For this review, use the dimensioned drawing (mm, ordinates from the lowest corner) and the shaded views. Round coordinates to 2 decimals unless told otherwise and drop trailing zeros. Loops run counter-clockwise (first coordinate to the right, second up) from the corner with the lowest first, then second, coordinate; pieces in that order, holes last. Notation, with made-up numbers: (-9, 35.25) -> (46, 35.25) arc R28 cw to (46, 55.25) -> close; hole circle Ø5 at (-31, -31.5). An arc over 180 degrees is marked (long way). Use one line per item in the form item = value. Start each with the question number.
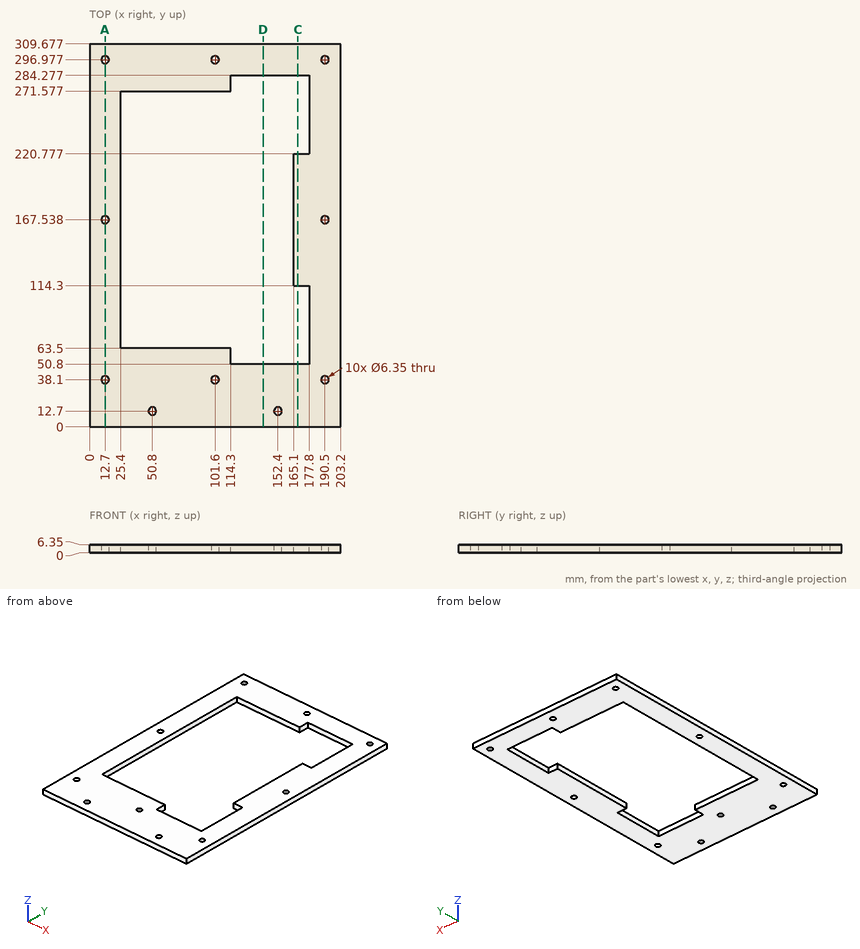
Item 1: Take a section at D-D on x = 140.5. Give the boundary of the cut face in (y, z), plus the area to 3 significant figures.
Item 2: Wall thickness on line 1 (Y direction, x = 190, z = 1) (1 decimal); line 2 (Y direction, x = 152.4, z = 4.25) (1 decimal); line 3 (Y direction, x = 101.6, z = 4.25) (1 decimal): over which ranges is each line inside the solid? List them lowest first.
Item 3: Take a section at A-A on x = 12.7. Give the number of separate pieces and of enclosed holes in the cut face.
Item 4: For P1, Ø5.5, axis at x = 190.5, y = 167.54, coming from the +Z side, flat-tipped, find the tip position at first contact; note if it passes through.
Item 5: Take a section at C-C on x = 168.5. Give the boundary of the cut face in (y, z), plus the area to 3 significant figures.
Results:
q1.outline = (0, 0) -> (50.8, 0) -> (50.8, 6.35) -> (0, 6.35) -> close; (284.28, 0) -> (309.68, 0) -> (309.68, 6.35) -> (284.28, 6.35) -> close
q1.area = 484 mm2
q2.line_1 = 0 to 35, 41.2 to 164.4, 170.7 to 293.8, 300.1 to 309.7
q2.line_2 = 0 to 9.5, 15.9 to 50.8, 284.3 to 309.7
q2.line_3 = 0 to 34.9, 41.3 to 63.5, 271.6 to 293.8, 300.2 to 309.7
q3.separate_pieces = 4
q3.enclosed_holes = 0
q4.P1 = through
q5.outline = (0, 0) -> (50.8, 0) -> (50.8, 6.35) -> (0, 6.35) -> close; (114.3, 0) -> (220.78, 0) -> (220.78, 6.35) -> (114.3, 6.35) -> close; (284.28, 0) -> (309.68, 0) -> (309.68, 6.35) -> (284.28, 6.35) -> close
q5.area = 1,160 mm2
